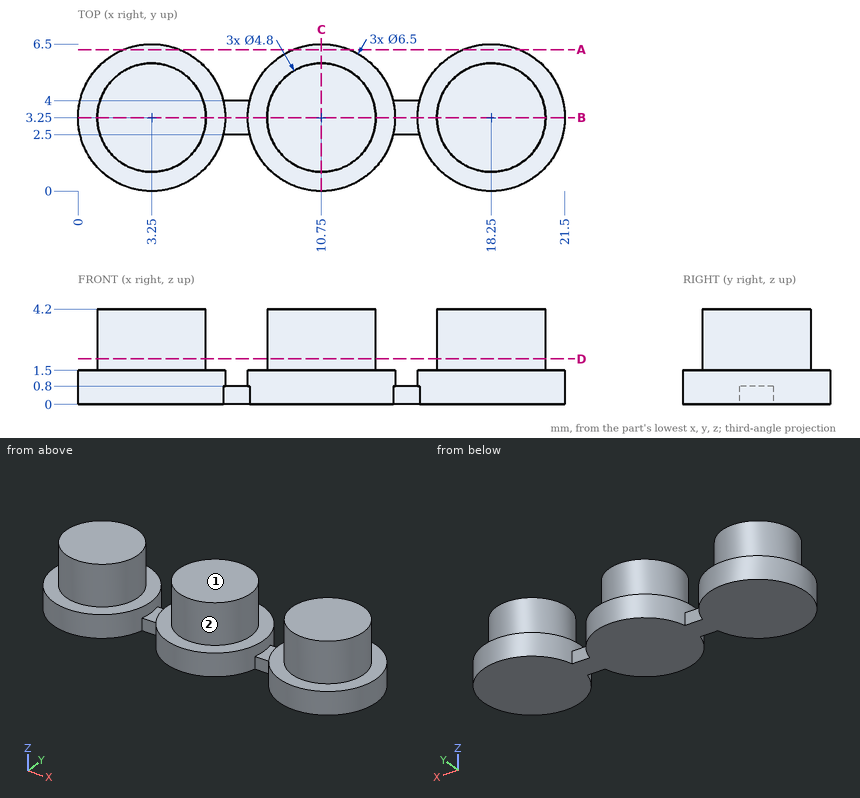
Answer from the drawing. Dimensions are ordinates in mm from the lowest x, y and z of the part. A direction names the side the tool comes from. Give positions to 0.01 mm unless a question says otherwise; leave off trailing zeros. Order: outer loops, then holes, each group sorted by start corner. A loop starts at its lowest first (then second) coordinate and runs counter-clockwise, first axis right, second up. Notation, with made-up numbers: (72.25, -9.5) -> (77.25, -9.5) arc R30 cw to (77.25, 20.5) -> close; hole circle Ø2 at (72, 42). An arc over 180 degrees is marked (long way). One line per item, written item: value. Start each with the question number.
(1) The part is cut by section C-C (x = 10.75). Determine the outline of the cut face in (y, z).
(2) The part is cut by section B-B (y = 3.25). Determine the outline of the cut face in (x, z).
(3) A tool of negligible diameter and unlimited length cuts with its end or side. For the marked faces 1 and 2, from which of +Z, -Z, +X, -X, +Y, -Y can it reach the whole face along a straight path? Write none if from no direction.
(4) Flat-ended cylindrical pins translate along their axes: P1, Ø1.5, axis at y = 2, z = 0.5, coming from the -X side; P2, Ø0.9, axis at x = 7, z = 0.5, coming from the +Y side; P3, Ø0.9, axis at x = 14.5, y = 3.5, coming from the +Z side. Find the tip coordinate at first contact, or state that the pin passes through.
(5) The part is cut by section D-D (z = 2). Determine the outline of the cut face in (x, y).
(6) Straight lines are drawn through the part: L1, parallel to X at y = 2.25, z = 3.75; L2, parallel to X at y = 3.5, z = 2.3; L3, parallel to Z at x = 11.25, y = 0.75. For each, find the intervals that lie inside material, in ascending order.
(7) The part is cut by section A-A (y = 6.25). Determine the outline of the cut face in (x, z).
Taken from the geometry:
1. outline: (0, 0) -> (6.5, 0) -> (6.5, 1.5) -> (5.65, 1.5) -> (5.65, 4.2) -> (0.85, 4.2) -> (0.85, 1.5) -> (0, 1.5) -> close
2. outline: (0, 0) -> (21.5, 0) -> (21.5, 1.5) -> (20.65, 1.5) -> (20.65, 4.2) -> (15.85, 4.2) -> (15.85, 1.5) -> (15, 1.5) -> (15, 0.8) -> (14, 0.8) -> (14, 1.5) -> (13.15, 1.5) -> (13.15, 4.2) -> (8.35, 4.2) -> (8.35, 1.5) -> (7.5, 1.5) -> (7.5, 0.8) -> (6.5, 0.8) -> (6.5, 1.5) -> (5.65, 1.5) -> (5.65, 4.2) -> (0.85, 4.2) -> (0.85, 1.5) -> (0, 1.5) -> close
3. face 1: +Z, +X, -X, +Y, -Y
3. face 2: +Z
4. P1: x = 0.04
4. P2: y = 4
4. P3: z = 0.8
5. outline: circle Ø4.8 at (3.25, 3.25); circle Ø4.8 at (10.75, 3.25); circle Ø4.8 at (18.25, 3.25)
6. L1: 1.07 to 5.43, 8.57 to 12.93, 16.07 to 20.43
6. L2: 0.86 to 5.64, 8.36 to 13.14, 15.86 to 20.64
6. L3: 0 to 1.5
7. outline: (2, 0) -> (4.5, 0) -> (4.5, 1.5) -> (2, 1.5) -> close; (9.5, 0) -> (12, 0) -> (12, 1.5) -> (9.5, 1.5) -> close; (17, 0) -> (19.5, 0) -> (19.5, 1.5) -> (17, 1.5) -> close
